```python
from build123d import *

# Parameters (mm, degrees)
BOSS_EXTRUDE1_DEPTH = 50
CUT_EXTRUDE1_DEPTH  = 48
FILLET1_R           = 1
FILLET2_R           = 2
SKETCH4_R           = 1.6
CUT_EXTRUDE2_DEPTH  = 2921.7864791


with BuildPart() as part:
    # Sketch2 → Boss-Extrude1 (new body)
    with BuildSketch(Plane.XY):
        with BuildLine():
            Line((2758.968126944, -672.549477124), (2746.968126944, -672.549477124))
            ThreePointArc((2746.968126944, -672.549477124), (2769.195793319, -726.211810748), (2822.858126944, -748.439477124))
            Line((2822.858126944, -748.439477124), (2822.858126944, -736.439477124))
            ThreePointArc((2822.858126944, -736.439477124), (2777.681074694, -717.726529374), (2758.968126944, -672.549477124))
        make_face()
    extrude(amount=BOSS_EXTRUDE1_DEPTH)

    # Sketch3 → Cut-Extrude1 (cut)
    with BuildSketch(Plane.XY.offset(50)):
        with BuildLine():
            Line((2756.968126944, -672.549477124), (2737.478838536, -672.549477124))
            Line((2737.478838536, -672.549477124), (2737.478838536, -757.577335174))
            Line((2737.478838536, -757.577335174), (2822.858126944, -757.577335174))
            Line((2822.858126944, -757.577335174), (2822.858126944, -738.439477124))
            ThreePointArc((2822.858126944, -738.439477124), (2776.266861131, -719.140742936), (2756.968126944, -672.549477124))
        make_face()
    extrude(amount=-CUT_EXTRUDE1_DEPTH, mode=Mode.SUBTRACT)

    # Fillet1
    fillet1_edges = [part.edges().sort_by_distance(p)[0] for p in [
        (2776.266861131, -719.140742936, 50),
        (2769.195793319, -726.211810748, 2),
    ]]
    fillet(fillet1_edges, radius=FILLET1_R)

    # Fillet2
    fillet2_edges = [part.edges().sort_by_distance(p)[0] for p in [
        (2776.266861131, -719.140742936, 2),
    ]]
    fillet(fillet2_edges, radius=FILLET2_R)

    # Sketch4 → Cut-Extrude2 (cut, through all)
    with BuildSketch(Plane.XY.offset(2)):
        with Locations((2802.858126944, -741.0807262)):
            Circle(SKETCH4_R)
        with Locations((2754.326877867, -692.549477124)):
            Circle(SKETCH4_R)
    extrude(amount=-CUT_EXTRUDE2_DEPTH, mode=Mode.SUBTRACT)


solid = part.part
```
Part model, mm, in its own coordinate system. A direction names the side the tool comes from. Coordinates: 2 decimals unless noted, no trailing zeros. Loops run counter-clockwise (first coordinate to the right, second up) from the corner with the lowest first, then second, coordinate; pieces in that order, holes last. Notation, with made-up numbers: (-7, 58.25) - (25, 58.25) arc R30 ccw to (25, 84.25) - close; hole circle Ø9 at (-22, -35). An arc over 180 degrees is marked (long way). Write item = value, one per line. Start each with the question number.
Item 1: 3-axis set-ups, long thin cutter, end or side, ignore diameter. For faces 1 (the cylindrical face through (2804.384, -740.6, 1.014)), 2 (the flat face through (2774, -721, 2)): which of +Z, -Z, +X, -X, +Y, -Y reach the whole face in a straight line?
Item 2: Cut at A-A, the plane z = 14. Give the cut face in (x, y), and give its area (3 significant figures).
Item 3: Flat gauge pins, fed straight in: pin 1 Ø1 at (y, z) = (-703, 29.5) entering from +X; pin 2 Ø2 at (y, z) = (-712.5, 20) entering from -X; pin 3 Ø8 at (x, z) = (2806, 41) entering from +Y. Where does each tip first touch, or does it go through?
Item 4: Wall check: L1, parallel to Z at x = 2815.5, y = -743; L2, parallel to X at y = -719, z = 17.5; L3, parallel to Y at x = 2795.5, z = 26.5. Give the ranges that are in metal, low to high. Write a range as from..to.
The answers:
q1.face_1 = +Z, -Z
q1.face_2 = +Z, -X, -Y
q2.outline = (2756.97, -672.55) arc R65.89 ccw to (2822.86, -738.44) - (2822.86, -736.44) arc R63.89 cw to (2758.97, -672.55) - close
q2.area = 204 mm2
q3.pin_1 = 2766.97
q3.pin_2 = 2769.71
q3.pin_3 = -732.94
q4.L1 = 0..2
q4.L2 = 2776.13..2778.99
q4.L3 = -732.49..-730.29
